Source: CAD feature listing. Evaluate the final solid. Frame: model axes, mm. Face numbers are marked on the shaded views. A direction names the side the tool comes from. Round coordinates to 2 decimals unless told otherwise and drop trailing zeros. Write each loop counter-clockwise with the first axis right and the second up, starting at its lowest first coordinate (ties: lowest second). Pieces come first, ordered by that corner, then holes. Notation, with made-up numbers: M 5.25,-11 L 22.25,-11 A31 cw 22.25,21 Z; hole C -37.75,72 d1. An arc over 180 degrees is marked long. Answer in a Markdown table with one row per item.
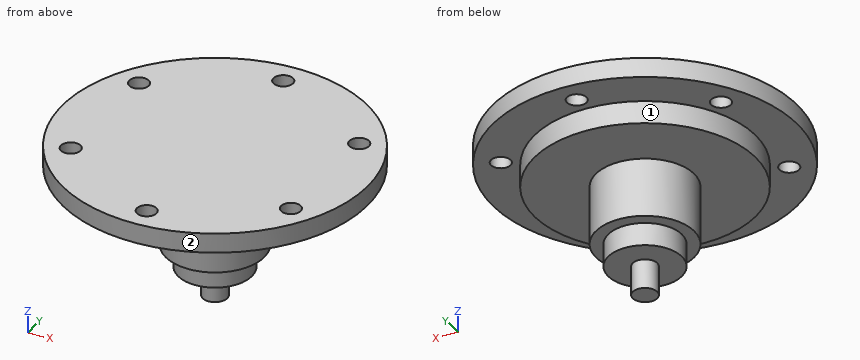
from build123d import *

# Parameters (mm, degrees)
SKETCH1_R           = 31
SKETCH1_R_2         = 2
BOSS_EXTRUDE1_DEPTH = 4
SKETCH2_R           = 22.5
BOSS_EXTRUDE2_DEPTH = 4.63
SKETCH3_R           = 10
BOSS_EXTRUDE3_DEPTH = 12
SKETCH4_R           = 7.5
BOSS_EXTRUDE4_DEPTH = 4.66
SKETCH7_R           = 2.505
BOSS_EXTRUDE5_DEPTH = 6


with BuildPart() as part:
    # Sketch1 → Boss-Extrude1 (new body)
    with BuildSketch(Plane.XY):
        Circle(SKETCH1_R)
        with Locations((0, 26)):
            Circle(SKETCH1_R_2, mode=Mode.SUBTRACT)
        with Locations((22.516660498, 13)):
            Circle(SKETCH1_R_2, mode=Mode.SUBTRACT)
        with Locations((22.516660498, -13)):
            Circle(SKETCH1_R_2, mode=Mode.SUBTRACT)
        with Locations((0, -26)):
            Circle(SKETCH1_R_2, mode=Mode.SUBTRACT)
        with Locations((-22.516660498, -13)):
            Circle(SKETCH1_R_2, mode=Mode.SUBTRACT)
        with Locations((-22.516660498, 13)):
            Circle(SKETCH1_R_2, mode=Mode.SUBTRACT)
    extrude(amount=BOSS_EXTRUDE1_DEPTH)

    # Sketch2 → Boss-Extrude2 (add)
    with BuildSketch(Plane(origin=(0, 0, 0), x_dir=(-1, 0, 0), z_dir=(0, 0, -1))):
        with Locations(Location((0, 0, 0), (0, 0, 180))):
            Circle(SKETCH2_R)
    extrude(amount=BOSS_EXTRUDE2_DEPTH)

    # Sketch3 → Boss-Extrude3 (add)
    with BuildSketch(Plane(origin=(0, 0, -4.63), x_dir=(-1, 0, 0), z_dir=(0, 0, -1))):
        Circle(SKETCH3_R)
    extrude(amount=BOSS_EXTRUDE3_DEPTH)

    # Sketch4 → Boss-Extrude4 (add)
    with BuildSketch(Plane(origin=(0, 0, -16.63), x_dir=(-1, 0, 0), z_dir=(0, 0, -1))):
        Circle(SKETCH4_R)
    extrude(amount=BOSS_EXTRUDE4_DEPTH)

    # Sketch7 → Boss-Extrude5 (add)
    with BuildSketch(Plane(origin=(0, 0, -21.29), x_dir=(-1, 0, 0), z_dir=(0, 0, -1))):
        Circle(SKETCH7_R)
    extrude(amount=BOSS_EXTRUDE5_DEPTH)


solid = part.part
Q1. Access query for the marked faces 1 and 2. Directions: +Z, -Z, +X, -X, +Y, -Y. A direction counts if a zero-diameter tool reaches every point of the face in a straight line with its end or side. Return the directions, or none.
Solutions:
| item | result |
|---|---|
| face 1 | -Z |
| face 2 | +Z, -Z |
Q2. Section D-D (z = -11.5). Return loops of the section in (x, y).
Solutions:
| item | result |
|---|---|
| outline | C 0,0 d20 |
Q3. Section B-B (y = -26). Return loops of the section in (x, z), and give its area (3 significant figures).
Solutions:
| item | result |
|---|---|
| outline | M -16.88,0 L -2,0 L -2,4 L -16.88,4 Z; M 2,0 L 16.88,0 L 16.88,4 L 2,4 Z |
| area | 119 mm2 |
Q4. Section A-A (x = 0). Return loops of the section in (y, z) (3 decimals), and give its area (3 significant figures).
Solutions:
| item | result |
|---|---|
| outline | M -31,0 L -28,0 L -28,4 L -31,4 Z; M -24,0 L -22.5,0 L -22.5,-4.63 L -10,-4.63 L -10,-16.63 L -7.5,-16.63 L -7.5,-21.29 L -2.505,-21.29 L -2.505,-27.29 L 2.505,-27.29 L 2.505,-21.29 L 7.5,-21.29 L 7.5,-16.63 L 10,-16.63 L 10,-4.63 L 22.5,-4.63 L 22.5,0 L 24,0 L 24,4 L -24,4 Z; M 28,0 L 31,0 L 31,4 L 28,4 Z |
| area | 764 mm2 |
Q5. Contact query for flat-ended pins moving along their axis: pin 1 Ø3 at (x, y) = (16, -12.5) entering from -Z; pin 2 Ø3 at (x, z) = (7, -12.5) entering from -Y; pin 3 Ø8 at (x, y) = (9, 3.5) entering from -Z; pin 4 Ø2.5 at (x, y) = (22.52, -13) entering from +Z. Output: stop coordinate, or through.
Solutions:
| item | result |
|---|---|
| pin 1 | stops at z = -4.63 |
| pin 2 | stops at y = -8.35 |
| pin 3 | stops at z = -21.29 |
| pin 4 | passes through |
Q6. Material intervals for probe 1 along Y at (x, z) = (0, 3.1); probe 2 along Z at (x, y) = (-2, 9); probe 3 along Z at (x, y) = (-13, -26), sorted ascending.
Solutions:
| item | result |
|---|---|
| probe 1 | y = -31 to -28, -24 to 24, 28 to 31 |
| probe 2 | z = -16.63 to 4 |
| probe 3 | z = 0 to 4 |
Q7. Section C-C (y = 13). Return loops of the section in (x, z), and give its area (3 significant figures).
Solutions:
| item | result |
|---|---|
| outline | M -28.14,0 L -24.52,0 L -24.52,4 L -28.14,4 Z; M -20.52,0 L -18.36,0 L -18.36,-4.63 L 18.36,-4.63 L 18.36,0 L 20.52,0 L 20.52,4 L -20.52,4 Z; M 24.52,0 L 28.14,0 L 28.14,4 L 24.52,4 Z |
| area | 363 mm2 |
